Can you work these out from the model? Positions are in its coordinate system, mm. Round coordinates to 2 decimals unless told otherwise and drop trailing zeros. Write each loop counter-clockwise with the first axis right and the second up, starting at its lowest first coordinate (ties: lowest second). Pieces come first, ordered by that corner, then holes. Notation, with made-up numbers: (23, -5.75) - (58, -5.75) arc R23 cw to (58, 7.25) - close; hole circle Ø6 at (32.25, 13). An arc over 180 degrees is marked (long way). One line per item, written item: value. Start each with the question number.
(1) Thinking about a two-plate mould opening in X: for faces 1 (the face through (-4, 0, 0.84)), 2 (the face through (-49.15, 0.74, 12.75)), 3 (the face through (-7.3, 18.6, 25)), which applies, +X half, -X half, draft (parallel to the pull), parting line (faces both ways), or undercut?
(2) I want a section at A-A on y = -22. List the corners of the cut face in (x, z) for me.
(3) I want a section at B-B on x = 6. List the corners of the cut face in (y, z) for me.
(4) I want a section at C-C on y = 15. List the corners of the cut face in (x, z) for me.
(5) If I drill on L1, parallel to X at y = 0, z = 18.75; L2, parallel to Y at x = -25, z = 8.5; L3, parallel to Z at x = 20.5, y = 5, over which ranges is the centre line in solid material (lowest first)? Write a range as from..to.
(6) I'm going to push flat-ended pins straight in: pin 1 Ø1.5 at (y, z) = (-19.5, 19.5) entering from -X; pin 2 Ø1.5 at (x, y) = (-16, 9.5) entering from +Z; pin 3 Ø5 at (x, z) = (26, 22.5) entering from +Y. Where does each tip first touch, or does it pass through?
from build123d import *

# Parameters (mm, degrees)
F1_DEPTH = 25
F2_R     = 12.6178924605
F3_T     = -0.84


with BuildPart() as f1:
    # F0 (on Top) → F1 (new body)
    with BuildSketch(Plane.XY):
        with BuildLine():
            ThreePointArc((-3.620624356, -12.9584835946), (-7.2412487119, 0), (-3.620624356, 12.9584835946))
            ThreePointArc((-3.620624356, 12.9584835946), (-50, 0), (-3.620624356, -12.9584835946))
        make_face()
        with BuildLine():
            ThreePointArc((-3.620624356, -12.9584835946), (-0.9221638109, -6.7273920987), (0, 0))
            ThreePointArc((0, 0), (-0.9221638109, 6.7273920987), (-3.620624356, 12.9584835946))
            ThreePointArc((-3.620624356, 12.9584835946), (-7.2412487119, 0), (-3.620624356, -12.9584835946))
        make_face()
        with BuildLine():
            ThreePointArc((-3.620624356, 12.9584835946), (-0.9221638109, 6.7273920987), (0, 0))
            ThreePointArc((0, 0), (-0.9221638109, -6.7273920987), (-3.620624356, -12.9584835946))
            ThreePointArc((-3.620624356, -12.9584835946), (24.4861433868, -24.0778361891), (42.7587512881, 0))
            ThreePointArc((42.7587512881, 0), (24.4861433868, 24.0778361891), (-3.620624356, 12.9584835946))
        make_face()
    extrude(amount=F1_DEPTH)

    # F2
    f2_edges = [f1.edges().sort_by_distance(p)[0] for p in [
        (-3.620624, 12.958484, 12.5),
        (-3.620624, -12.958484, 12.5),
    ]]
    fillet(f2_edges, radius=F2_R)

    # F3
    f3_openings = [f1.faces().sort_by_distance(p)[0] for p in [
        (-3.620624, 0, 25),
    ]]
    offset(amount=F3_T, openings=f3_openings, kind=Kind.INTERSECTION)


solid = f1.part
Established:
1. face 1: undercut
1. face 2: undercut
1. face 3: draft
2. outline: (-36.87, 0) - (-13.13, 0) - (-13.13, 25) - (-15.01, 25) - (-15.01, 0.84) - (-34.99, 0.84) - (-34.99, 25) - (-36.87, 25) - close; (5.88, 0) - (29.63, 0) - (29.63, 25) - (27.74, 25) - (27.74, 0.84) - (7.77, 0.84) - (7.77, 25) - (5.88, 25) - close
3. outline: (-22.06, 0) - (22.06, 0) - (22.06, 25) - (21.11, 25) - (21.11, 0.84) - (-21.11, 0.84) - (-21.11, 25) - (-22.06, 25) - close
4. outline: (-45, 0) - (37.76, 0) - (37.76, 25) - (36.7, 25) - (36.7, 0.84) - (-43.94, 0.84) - (-43.94, 25) - (-45, 25) - close
5. L1: -50..-49.16, 41.92..42.76
5. L2: -25..-24.16, 24.16..25
5. L3: 0..0.84
6. pin 1: x = -41.54
6. pin 2: z = 0.84
6. pin 3: y = 24.33
